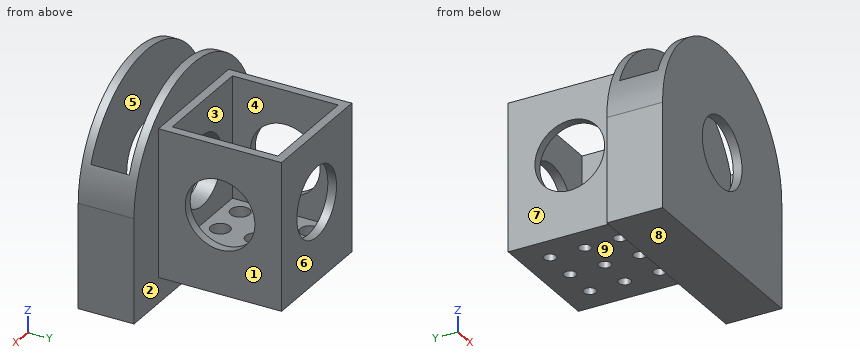
from build123d import *

# Parameters (mm, degrees)
SKETCH1_W                 = 44.85
SKETCH1_H                 = 44.85
SKETCH1_W_2               = 38.5
SKETCH1_H_2               = 38.5
BOSS_EXTRUDE1_DEPTH       = 19.25
SKETCH2_W                 = 44.85
SKETCH2_H                 = 44.85
BOSS_EXTRUDE2_DEPTH       = 3.175
SKETCH3_W                 = 44.85
SKETCH3_H                 = 44.85
BOSS_EXTRUDE3_DEPTH       = 3.175
SKETCH5_R                 = 12.7
CUT_EXTRUDE1_DEPTH        = 3.175
SKETCH8_W                 = 44.85
SKETCH8_H                 = 44.85
SKETCH8_R                 = 2.2225
BOSS_EXTRUDE4_DEPTH       = 6.35
SKETCH9_R                 = 3.4925
CUT_EXTRUDE4_DEPTH        = 6.35
CUT_EXTRUDE5_REACH        = 62.226
SKETCH10_W                = 38.5
SKETCH10_H                = 38.5
SKETCH15_W                = 44.85
SKETCH15_H                = 44.85
SKETCH15_W_2              = 38.5
SKETCH15_H_2              = 38.5
BOSS_EXTRUDE8_DEPTH       = 2.575
CUT_EXTRUDE3_DEPTH        = 43.822445925
CUT_EXTRUDE3_DEPTH_BACK   = 43.822445925
SKETCH7_R                 = 12.7
SKETCH16_R                = 38.1
BOSS_EXTRUDE9_DEPTH       = 20.32
CUT_EXTRUDE2_DEPTH        = 69.777576469
CUT_EXTRUDE2_DEPTH_BACK   = 69.777576469
SKETCH6_R                 = 12.7
CUT_EXTRUDE6_START        = -3.175
CUT_EXTRUDE6_DEPTH        = 13.97
BOSS_EXTRUDE10_REACH      = 108.878
BOSS_EXTRUDE10_END_RADIUS = 38.1
BOSS_EXTRUDE10_START      = -38.1
SKETCH18_W                = 76.2
SKETCH18_H                = 20.32


with BuildPart() as part:
    # Sketch1 → Boss-Extrude1 (new, symmetric)
    with BuildSketch(Plane(origin=(0, 0, 0), x_dir=(1, 0, 0), z_dir=(0, 1, 0))):
        Rectangle(SKETCH1_W, SKETCH1_H)
        Rectangle(SKETCH1_W_2, SKETCH1_H_2, mode=Mode.SUBTRACT)
    extrude(amount=BOSS_EXTRUDE1_DEPTH, both=True)

    # Sketch2 → Boss-Extrude2 (add)
    with BuildSketch(Plane(origin=(0, 19.25, 0), x_dir=(1, 0, 0), z_dir=(0, 1, 0))):
        Rectangle(SKETCH2_W, SKETCH2_H)
    extrude(amount=BOSS_EXTRUDE2_DEPTH)

    # Sketch3 → Boss-Extrude3 (add)
    with BuildSketch(Plane.XZ.offset(19.25)):
        Rectangle(SKETCH3_W, SKETCH3_H)
    extrude(amount=BOSS_EXTRUDE3_DEPTH)

    # Sketch5 → Cut-Extrude1 (cut)
    with BuildSketch(Plane(origin=(0, -22.425, -22.425), x_dir=(1, 0, 0), z_dir=(0, 1, 0))):
        with Locations(Location((0, -22.425, 0), (0, 0, 90))):
            Circle(SKETCH5_R)
    extrude(amount=CUT_EXTRUDE1_DEPTH, mode=Mode.SUBTRACT)

    # Sketch8 → Boss-Extrude4 (add)
    with BuildSketch(Plane(origin=(0, 0, -22.425), x_dir=(-1, 0, 0), z_dir=(0, 0, -1))):
        Rectangle(SKETCH8_W, SKETCH8_H)
        with Locations((-12.7, 12.7)):
            Circle(SKETCH8_R, mode=Mode.SUBTRACT)
        with Locations((0, 12.7)):
            Circle(SKETCH8_R, mode=Mode.SUBTRACT)
        with Locations((12.7, 12.7)):
            Circle(SKETCH8_R, mode=Mode.SUBTRACT)
        Circle(SKETCH8_R, mode=Mode.SUBTRACT)
        with Locations((12.7, 0)):
            Circle(SKETCH8_R, mode=Mode.SUBTRACT)
        with Locations((0, -12.7)):
            Circle(SKETCH8_R, mode=Mode.SUBTRACT)
        with Locations((12.7, -12.7)):
            Circle(SKETCH8_R, mode=Mode.SUBTRACT)
        with Locations((-12.7, 0)):
            Circle(SKETCH8_R, mode=Mode.SUBTRACT)
        with Locations((-12.7, -12.7)):
            Circle(SKETCH8_R, mode=Mode.SUBTRACT)
    extrude(amount=BOSS_EXTRUDE4_DEPTH)

    # Sketch9 → Cut-Extrude4 (cut)
    with BuildSketch(Plane.XY.offset(-19.25)):
        with Locations((12.7, 12.7)):
            Circle(SKETCH9_R)
        with Locations((0, 12.7)):
            Circle(SKETCH9_R)
        with Locations((-12.7, 12.7)):
            Circle(SKETCH9_R)
        Circle(SKETCH9_R)
        with Locations((-12.7, 0)):
            Circle(SKETCH9_R)
        with Locations((0, -12.7)):
            Circle(SKETCH9_R)
        with Locations((-12.7, -12.7)):
            Circle(SKETCH9_R)
        with Locations((12.7, 0)):
            Circle(SKETCH9_R)
        with Locations((12.7, -12.7)):
            Circle(SKETCH9_R)
    extrude(amount=-CUT_EXTRUDE4_DEPTH, mode=Mode.SUBTRACT)

    # Sketch10 → Cut-Extrude5 (cut, up to next)
    with BuildSketch(Plane.XY.offset(22.425), mode=Mode.PRIVATE) as cut_extrude5_sk1:
        Rectangle(SKETCH10_W, SKETCH10_H)
    cut_extrude5_tool1 = extrude(cut_extrude5_sk1.sketch, amount=-CUT_EXTRUDE5_REACH, mode=Mode.PRIVATE) & part.part
    add(cut_extrude5_tool1.solids().sort_by_distance((0, 0, 22.425))[0], mode=Mode.SUBTRACT)

    # Sketch15 → Boss-Extrude8 (add)
    with BuildSketch(Plane.XY.offset(22.425)):
        Rectangle(SKETCH15_W, SKETCH15_H)
        Rectangle(SKETCH15_W_2, SKETCH15_H_2, mode=Mode.SUBTRACT)
    extrude(amount=BOSS_EXTRUDE8_DEPTH)

    # Sketch7 → Cut-Extrude3 (cut, two sides: drawn at the far end of the back side and taken through both)
    with BuildSketch(Plane.ZY.offset(-CUT_EXTRUDE3_DEPTH_BACK)):
        with Locations(Location((0, 0, 0), (0, 0, 180))):
            Circle(SKETCH7_R)
    extrude(amount=CUT_EXTRUDE3_DEPTH + CUT_EXTRUDE3_DEPTH_BACK, mode=Mode.SUBTRACT)

    # Sketch16 → Boss-Extrude9 (add)
    with BuildSketch(Plane.XZ.offset(22.425)):
        with Locations(Location((0, 0, 0), (0, 0, 270))):
            Circle(SKETCH16_R)
    extrude(amount=BOSS_EXTRUDE9_DEPTH)

    # Sketch6 → Cut-Extrude2 (cut, two sides: drawn at the far end of the back side and taken through both)
    with BuildSketch(Plane(origin=(0, 0, 0), x_dir=(1, 0, 0), z_dir=(0, 1, 0)).offset(-CUT_EXTRUDE2_DEPTH_BACK)):
        with Locations(Location((0, 0, 0), (0, 0, 90))):
            Circle(SKETCH6_R)
    extrude(amount=CUT_EXTRUDE2_DEPTH + CUT_EXTRUDE2_DEPTH_BACK, mode=Mode.SUBTRACT)

    # Sketch17 → Cut-Extrude6 (cut)
    with BuildSketch(Plane.XZ.offset(42.745).offset(CUT_EXTRUDE6_START)):
        with BuildLine():
            Line((-35.56, 0), (-35.56, 38.1))
            Line((-35.56, 38.1), (35.56, 38.1))
            Line((35.56, 38.1), (35.56, 0))
            ThreePointArc((35.56, 0), (0, -35.56), (-35.56, 0))
        make_face()
    extrude(amount=-CUT_EXTRUDE6_DEPTH, mode=Mode.SUBTRACT)

    # Boss-Extrude10: up to this cylinder (the profile starts outside it)
    boss_extrude10_end = Plane(origin=(0, -32.585, 0), z_dir=(0, 1, 0)) * Cylinder(BOSS_EXTRUDE10_END_RADIUS, 294.956, mode=Mode.PRIVATE)
    # Sketch18 → Boss-Extrude10 (add, up to the surface)
    with BuildSketch(Plane.XY.offset(BOSS_EXTRUDE10_START), mode=Mode.PRIVATE) as boss_extrude10_sk1:
        with Locations((0, -32.585)):
            Rectangle(SKETCH18_W, SKETCH18_H)
    boss_extrude10_tool1 = extrude(boss_extrude10_sk1.sketch, amount=BOSS_EXTRUDE10_REACH, mode=Mode.PRIVATE) - boss_extrude10_end
    add(boss_extrude10_tool1.solids().sort_by_distance((0, -32.585, -38.1))[0])
    add(boss_extrude10_tool1.solids().sort_by_distance((0, -32.585, -38.1))[1])


solid = part.part
Can you work these out from the model? Positions are in its coordinate system, mm. Face numbers are marked on the shaded views. A direction names the side the tool comes from. Give positions to 0.01 mm unless a question says otherwise; leave off trailing zeros. Loops run counter-clockwise (first coordinate to the right, second up) from the corner with the lowest first, then second, coordinate; pieces in that order, holes last. Notation, with made-up numbers: (37.25, -30) -> (67.25, -30) arc R18 ccw to (67.25, 1) -> close; hole circle Ø4 at (-36.5, 85.5). An arc over 180 degrees is marked (long way). Use one line per item in the form item = value.
1) For the marked faces 5, 6, 7, 8 and 9, which set-ups out of +Z, -Z, +X, -X, +Y, -Y let a thin tool reach every point of the face, with its end or its side?
Answers:
face_5 = +Z
face_6 = +Z, -Z, +X, -X, +Y
face_7 = +Z, -Z, -X, +Y
face_8 = -Z, +X, -X, +Y, -Y
face_9 = -Z, +X, -X, +Y
2) If we section it at B-B (y = 8): Please give me the cut outline in (x, z) (3 decimals).
Answers:
outline = (-22.425, -28.775) -> (22.425, -28.775) -> (22.425, -9.864) -> (19.25, -9.864) -> (19.25, -19.25) -> (-19.25, -19.25) -> (-19.25, -9.864) -> (-22.425, -9.864) -> close; (-22.425, 9.864) -> (-19.25, 9.864) -> (-19.25, 25) -> (-22.425, 25) -> close; (19.25, 9.864) -> (22.425, 9.864) -> (22.425, 25) -> (19.25, 25) -> close
3) Will these pins go through, and if not, where does the flat tip stop? pin 1 (6 mm diameter, centred on x = -28.5, z = 6, fed in from +Y) (3 decimals); pin 2 (6 mm diameter, centred on y = 7.5, z = -26.5, fed in from +X) (3 decimals); pin 3 (3 mm diameter, centred on x = 18.5, y = -27.5, fed in from +Z); pin 4 (3.5 mm diameter, centred on x = 0, y = -12.5, fed in from +Z).
Answers:
pin_1 = -22.425
pin_2 = 22.425
pin_3 = -29.4
pin_4 = through
4) If we section it at A-A (z = -24.5): Count the separate pieces of the cut face and the enclosed holes in it, plus the area to 3 significant figures.
Answers:
separate_pieces = 1
enclosed_holes = 10
area = 2,490 mm²
5) We'd pull the mould along Y, two halves only. Please class the marked faces 1, 2, 3 and 4: released by +Y, released by -Y, zero draft, split by the parting line, or undercut.
Answers:
face_1 = zero draft
face_2 = released by +Y
face_3 = undercut
face_4 = undercut
6) I need wall thicknesses on line 1 along Y through (x, z) = (0, -27.1) (1 decimal); line 2 along Y through (x, z) = (-12.7, -21) (1 decimal); line 3 along Y through (x, z) = (13.5, -5) (3 decimals). Which ranges of each line are inside material? Lowest first, please.
Answers:
line_1 = -42.7 to -39.6, -25.6 to -14.9, -10.5 to -2.2, 2.2 to 10.5, 14.9 to 22.4
line_2 = -42.7 to -39.6, -25.6 to -16.2, -9.2 to -3.5, 3.5 to 9.2, 16.2 to 22.4
line_3 = -42.745 to -39.57, -25.6 to -19.25, 19.25 to 22.425
7) If we section it at D-D (y = -32): Please give me the cut outline in (x, z), plus the area to 3 significant figures.
Answers:
outline = (-38.1, -38.1) -> (38.1, -38.1) -> (38.1, 0) arc R38.1 ccw to (35.56, 13.68) -> (35.56, 0) arc R35.56 cw to (-35.56, 0) -> (-35.56, 13.68) arc R38.1 ccw to (-38.1, 0) -> close
area = 964 mm²
